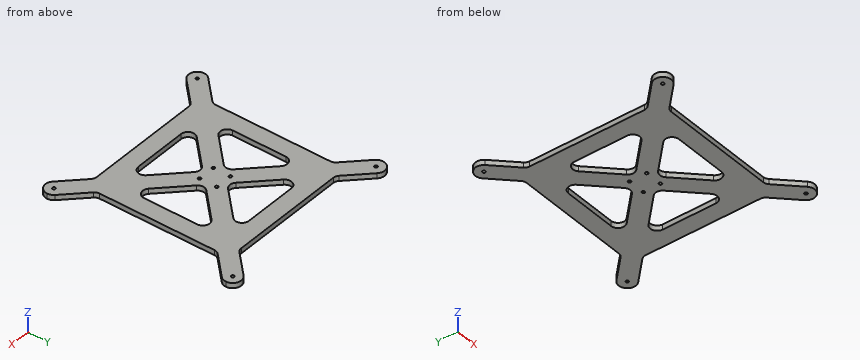
from build123d import *

# Parameters (mm, degrees)
F0_R     = 1.725
F1_DEPTH = 6
F2_R     = 8


with BuildPart() as f1:
    # F0 (on Top) → F1 (new body)
    with BuildSketch(Plane.XY):
        with BuildLine():
            ThreePointArc((-7.0710678119, 201.9289321881), (3.8268343237, 199.7612046749), (10, 209))
            ThreePointArc((10, 209), (9.2387953251, 212.8268343237), (7.0710678119, 216.0710678119))
            ThreePointArc((7.0710678119, 216.0710678119), (-7.0710678119, 216.0710678119), (-7.0710678119, 201.9289321881))
        make_face()
        with Locations((0, 209)):
            Circle(F0_R, mode=Mode.SUBTRACT)
        with BuildLine():
            ThreePointArc((7.0710678119, 216.0710678119), (9.2387953251, 212.8268343237), (10, 209))
            ThreePointArc((10, 209), (3.8268343237, 199.7612046749), (-7.0710678119, 201.9289321881))
            Line((-7.0710678119, 201.9289321881), (20, 174.8578643763))
            Line((20, 174.8578643763), (40, 154.8578643763))
            Line((40, 154.8578643763), (90.3578643763, 104.5))
            Line((90.3578643763, 104.5), (104.5, 118.6421356237))
            Line((104.5, 118.6421356237), (54.1421356237, 169))
            Line((54.1421356237, 169), (34.1421356237, 189))
            Line((34.1421356237, 189), (7.0710678119, 216.0710678119))
        make_face()
        with Locations((94.5, 114.5)):
            Circle(F0_R, mode=Mode.SUBTRACT)
        Polygon((174.8578643763, 189), (34.1421356237, 189), (54.1421356237, 169), (154.8578643763, 169), align=None)
        Polygon((40, 154.8578643763), (20, 174.8578643763), (20, 34.1421356237), (40, 54.1421356237), align=None)
        with BuildLine():
            Line((201.9289321881, 216.0710678119), (174.8578643763, 189))
            Line((174.8578643763, 189), (154.8578643763, 169))
            Line((154.8578643763, 169), (104.5, 118.6421356237))
            Line((104.5, 118.6421356237), (118.6421356237, 104.5))
            Line((118.6421356237, 104.5), (169, 154.8578643763))
            Line((169, 154.8578643763), (189, 174.8578643763))
            Line((189, 174.8578643763), (216.0710678119, 201.9289321881))
            ThreePointArc((216.0710678119, 201.9289321881), (201.9289321881, 201.9289321881), (201.9289321881, 216.0710678119))
        make_face()
        with Locations((114.5, 114.5)):
            Circle(F0_R, mode=Mode.SUBTRACT)
        with BuildLine():
            Line((40, 54.1421356237), (20, 34.1421356237))
            Line((20, 34.1421356237), (-7.0710678119, 7.0710678119))
            ThreePointArc((-7.0710678119, 7.0710678119), (3.8268343237, 9.2387953251), (10, 0))
            ThreePointArc((10, 0), (9.2387953251, -3.8268343237), (7.0710678119, -7.0710678119))
            Line((7.0710678119, -7.0710678119), (34.1421356237, 20))
            Line((34.1421356237, 20), (54.1421356237, 40))
            Line((54.1421356237, 40), (104.5, 90.3578643763))
            Line((104.5, 90.3578643763), (90.3578643763, 104.5))
            Line((90.3578643763, 104.5), (40, 54.1421356237))
        make_face()
        with Locations((94.5, 94.5)):
            Circle(F0_R, mode=Mode.SUBTRACT)
        with BuildLine():
            ThreePointArc((219, 209), (212.8268343237, 218.2387953251), (201.9289321881, 216.0710678119))
            ThreePointArc((201.9289321881, 216.0710678119), (201.9289321881, 201.9289321881), (216.0710678119, 201.9289321881))
            ThreePointArc((216.0710678119, 201.9289321881), (218.2387953251, 205.1731656763), (219, 209))
        make_face()
        with Locations((209, 209)):
            Circle(F0_R, mode=Mode.SUBTRACT)
        with BuildLine():
            ThreePointArc((10, 0), (3.8268343237, 9.2387953251), (-7.0710678119, 7.0710678119))
            ThreePointArc((-7.0710678119, 7.0710678119), (-7.0710678119, -7.0710678119), (7.0710678119, -7.0710678119))
            ThreePointArc((7.0710678119, -7.0710678119), (9.2387953251, -3.8268343237), (10, 0))
        make_face()
        Circle(F0_R, mode=Mode.SUBTRACT)
        with BuildLine():
            Line((169, 54.1421356237), (118.6421356237, 104.5))
            Line((118.6421356237, 104.5), (104.5, 90.3578643763))
            Line((104.5, 90.3578643763), (154.8578643763, 40))
            Line((154.8578643763, 40), (174.8578643763, 20))
            Line((174.8578643763, 20), (201.9289321881, -7.0710678119))
            ThreePointArc((201.9289321881, -7.0710678119), (201.9289321881, 7.0710678119), (216.0710678119, 7.0710678119))
            Line((216.0710678119, 7.0710678119), (189, 34.1421356237))
            Line((189, 34.1421356237), (169, 54.1421356237))
        make_face()
        with Locations((114.5, 94.5)):
            Circle(F0_R, mode=Mode.SUBTRACT)
        Polygon((169, 154.8578643763), (169, 54.1421356237), (189, 34.1421356237), (189, 174.8578643763), align=None)
        Polygon((174.8578643763, 20), (154.8578643763, 40), (54.1421356237, 40), (34.1421356237, 20), align=None)
        with BuildLine():
            ThreePointArc((219, 0), (218.2387953251, 3.8268343237), (216.0710678119, 7.0710678119))
            ThreePointArc((216.0710678119, 7.0710678119), (201.9289321881, 7.0710678119), (201.9289321881, -7.0710678119))
            ThreePointArc((201.9289321881, -7.0710678119), (212.8268343237, -9.2387953251), (219, 0))
        make_face()
        with Locations((209, 0)):
            Circle(F0_R, mode=Mode.SUBTRACT)
        Polygon((118.6421356237, 104.5), (104.5, 118.6421356237), (90.3578643763, 104.5), (104.5, 90.3578643763), align=None)
    extrude(amount=F1_DEPTH)

    # F2
    f2_edges = [f1.edges().sort_by_distance(p)[0] for p in [
        (20, 174.857864, 3),
        (20, 34.142136, 3),
        (34.142136, 20, 3),
        (174.857864, 20, 3),
        (189, 174.857864, 3),
        (189, 34.142136, 3),
        (174.857864, 189, 3),
        (34.142136, 189, 3),
        (104.5, 118.642136, 3),
        (154.857864, 169, 3),
        (90.357864, 104.5, 3),
        (104.5, 90.357864, 3),
        (169, 154.857864, 3),
        (54.142136, 169, 3),
        (118.642136, 104.5, 3),
        (40, 54.142136, 3),
        (54.142136, 40, 3),
        (154.857864, 40, 3),
        (169, 54.142136, 3),
        (40, 154.857864, 3),
    ]]
    fillet(f2_edges, radius=F2_R)


solid = f1.part
Source: CAD feature listing. Evaluate the final solid. Frame: model axes, mm. Give positions to 0.01 mm unless a question says otherwise; leave off trailing zeros. Order: outer loops, then holes, each group sorted by start corner. A loop starts at its lowest first (then second) coordinate and runs counter-clockwise, first axis right, second up. Notation, with made-up numbers: (18.25, 84) -> (22.25, 84) arc R10 cw to (22.25, 88) -> close; hole circle Ø1 at (23.5, -11). An arc over 180 degrees is marked (long way). Write item = value, one per line.
Item 1: Contact query for flat-ended pins moving along their axis: pin 1 (2 mm diameter, centred on x = 209, y = 209, fed in from -Z); pin 2 (1 mm diameter, centred on x = 89, z = 1.5, fed in from -Y); pin 3 (2 mm diameter, centred on x = 23.5, z = 3, fed in from +Y); pin 4 (2 mm diameter, centred on y = 64, z = 2, fed in from -X). Output: stop coordinate, or through.
Check result:
pin_1 = through
pin_2 = 20
pin_3 = 200.64
pin_4 = 20
Item 2: Section query C-C (y = 82). Output: boundary loops of the cut face in (x, z).
Check result:
outline = (20, 0) -> (40, 0) -> (40, 6) -> (20, 6) -> close; (67.86, 0) -> (96.14, 0) -> (96.14, 6) -> (67.86, 6) -> close; (112.86, 0) -> (141.14, 0) -> (141.14, 6) -> (112.86, 6) -> close; (169, 0) -> (189, 0) -> (189, 6) -> (169, 6) -> close
Item 3: Ray query, probe 1 along Y at (x, z) = (104.5, 5.7); probe 2 along X at (y, z) = (114.5, 3.6) (3 decimals); probe 3 along Y at (x, z) = (128, 3.1). Return the intervals inside material, ascending.
Check result:
probe_1 = 20 to 40, 87.04 to 121.96, 169 to 189
probe_2 = 20 to 40, 80.358 to 92.775, 96.225 to 112.775, 116.225 to 128.642, 169 to 189
probe_3 = 20 to 40, 66.86 to 95.14, 113.86 to 142.14, 169 to 189
Item 4: Section query B-B (z = 3.1). State how many separate pieces and enclosed holes the cut face has, then the cut area to 3 significant figures.
Check result:
separate_pieces = 1
enclosed_holes = 12
area = 22,300 mm²
Item 5: Section query D-D (y = 45.5). Output: boundary loops of the cut face in (x, z), then the cut area to 3 significant figures.
Check result:
outline = (20, 0) -> (65.86, 0) -> (65.86, 6) -> (20, 6) -> close; (143.14, 0) -> (189, 0) -> (189, 6) -> (143.14, 6) -> close
area = 550 mm²
Item 6: Section query A-A (y = 165.5). Output: boundary loops of the cut face in (x, z), then the cut area to 3 significant figures.
Check result:
outline = (20, 0) -> (66.84, 0) -> (66.84, 6) -> (20, 6) -> close; (142.16, 0) -> (189, 0) -> (189, 6) -> (142.16, 6) -> close
area = 562 mm²
